```python
from build123d import *

# Parameters (mm, degrees)
F1_DEPTH  = 12.7
F2_R      = 6.35
F3_DEPTH  = 31.242
F4_W      = 6.35
F4_H      = 38.1
F5_DEPTH  = 38.1
F7_DEPTH  = 61.468
F9_DEPTH  = 25.4
F10_R     = 3.175
F11_DEPTH = 50.8


with BuildPart() as f1:
    # F0 (on Top) → F1 (new body)
    with BuildSketch(Plane.XY):
        with BuildLine():
            Line((12.7, -30.8671), (12.697872, 45.100048))
            ThreePointArc((12.697872, 45.100048), (-0.230077, 58.03046), (-12.681114, 44.640199))
            Line((-12.681114, 44.640199), (-12.681114, -30.175112))
            Line((-12.681114, -30.175112), (-12.681114, -31.559801))
            ThreePointArc((-12.681114, -31.559801), (0.346479, -43.562729), (12.7, -30.8671))
        make_face()
        with BuildLine():
            Line((-12.681114, -31.559801), (-12.681114, -30.175112))
            ThreePointArc((-12.681114, -30.175112), (-12.7, -30.867456), (-12.681114, -31.559801))
        make_face()
    extrude(amount=F1_DEPTH)

    # F2 (on face) → F3 (cut)
    with BuildSketch(Plane.XY.offset(12.7)):
        with Locations((0, -30.867456)):
            Circle(F2_R)
        with Locations((0, 45.332544)):
            Circle(F2_R)
    extrude(amount=-F3_DEPTH, mode=Mode.SUBTRACT)

    # F4 (on face) → F5 (join)
    with BuildSketch(Plane.XY.offset(12.7)):
        with Locations((3.175, 7.232544)):
            Rectangle(F4_W, F4_H)
        with Locations((-3.175, 7.232544)):
            Rectangle(F4_W, F4_H)
    extrude(amount=F5_DEPTH)

    # F6 (on face) → F7 (cut)
    with BuildSketch(Plane.XZ.offset(11.817456)):
        with BuildLine():
            ThreePointArc((-6.35, 44.45), (-4.490128, 48.940128), (0, 50.8))
            Line((0, 50.8), (-6.35, 50.8))
            Line((-6.35, 50.8), (-6.35, 44.45))
        make_face()
        with BuildLine():
            ThreePointArc((0, 50.8), (4.490128, 48.940128), (6.35, 44.45))
            Line((6.35, 44.45), (6.35, 50.8))
            Line((6.35, 50.8), (0, 50.8))
        make_face()
    extrude(amount=-F7_DEPTH, mode=Mode.SUBTRACT)

    # F8 (on face) → F9 (cut)
    with BuildSketch(Plane.YZ.offset(6.35)):
        with BuildLine():
            Line((-2.292456, 44.45), (-2.292456, 28.575))
            ThreePointArc((-2.292456, 28.575), (7.32078, 19.050409), (16.755909, 28.751465))
            Line((16.755909, 28.751465), (16.755909, 53.781159))
            Line((16.755909, 53.781159), (-2.292456, 53.781159))
            Line((-2.292456, 53.781159), (-2.292456, 44.45))
        make_face()
    extrude(amount=-F9_DEPTH, mode=Mode.SUBTRACT)

    # F10 (on face) → F11 (cut)
    with BuildSketch(Plane.XZ.offset(11.817456)):
        with Locations((0, 44.45)):
            Circle(F10_R)
    extrude(amount=-F11_DEPTH, mode=Mode.SUBTRACT)


solid = f1.part
```
Source: CAD feature listing. Evaluate the final solid. Frame: model axes, mm. A direction names the side the tool comes from. Round coordinates to 2 decimals unless told otherwise and drop trailing zeros. Loops run counter-clockwise (first coordinate to the right, second up) from the corner with the lowest first, then second, coordinate; pieces in that order, holes last. Notation, with made-up numbers: M -31.75,82 L 1.25,82 A18 cw 1.25,101 Z; hole C -17,15 d7. An arc over 180 degrees is marked long. Use a Markdown table: item, result. Add a question column.
1. Mould query, pull axis X, two halves, no side actions, for faces 1 (the cylindrical face through (-0.83, 51.63, 6.44)), 2 (the flat face through (-6.35, 7, 18)), 3 (the flat face through (0, 26.283, 31)). Classes: pulls with the +X half, pulls with the -X half, needs draft (parallel to the pull), parting line crosses it, or undercut.
2. Section query D-D on x = 7.5. Return the cut outline in (y, z), then the cut area to 3 significant figures.
3. Reachability of faces 4 (the flat face through (0, -11.817, 31)), 5 (the flat face through (6.35, 7, 18)), 6 (the flat face through (0, 16.756, 37)) from +Z, -Z, +X, -X, +Y, -Y: full face, straight path, thin tool, end or side. Return the list, or none.
4. Line query: line 1 (Y direction, x = -2, z = 48.5); line 2 (Y direction, x = 2, z = 12.5); line 3 (X direction, y = -8.5, z = 3). Output: solid intervals per line, ascending.
5. Section query C-C on y = 21.5. Return the cut outline in (x, z) (3 decimals).
6. Section query B-B on y = 47.5. Return the cut outline in (x, z).
7. Section query A-A on z = 32.5. Return the cut outline in (x, y).
8. Contact query for flat-ended pins moving along their axis: P1, Ø4, axis at x = 0, z = 35.5, coming from the -Y side; P2, Ø6.5, axis at y = 21.5, z = 6.5, coming from the -X side; P3, Ø12, axis at x = -8.5, z = 17.5, coming from the -Y side. Output: stop coordinate, or through.
Reported:
| question | item | result |
|---|---|---|
| 1 | face 1 | undercut |
| 1 | face 2 | pulls with the -X half |
| 1 | face 3 | needs draft |
| 2 | outline | M -41.12,0 L 55.58,0 L 55.58,12.7 L -41.12,12.7 Z |
| 2 | area | 1,230 mm² |
| 3 | face 4 | +Z, +X, -X, -Y |
| 3 | face 5 | +Z, +X, +Y, -Y |
| 3 | face 6 | +Z, +X, -X |
| 4 | line 1 | y = -11.82 to -2.29, 16.76 to 26.28 |
| 4 | line 2 | y = -43.41 to -36.89, -24.84 to 39.31, 51.36 to 57.87 |
| 4 | line 3 | x = -12.68 to 12.7 |
| 5 | outline | M -12.681,0 L 12.699,0 L 12.699,12.7 L 6.35,12.7 L 6.35,44.45 A6.35 ccw -6.35,44.45 L -6.35,12.7 L -12.681,12.7 Z; hole C 0,44.45 d6.35 |
| 6 | outline | M -12.51,0 L -5.97,0 L -5.97,12.7 L -12.51,12.7 Z; M 5.97,0 L 12.51,0 L 12.51,12.7 L 5.97,12.7 Z |
| 7 | outline | M -6.35,-11.82 L 6.35,-11.82 L 6.35,-2.29 L -6.35,-2.29 Z; M -6.35,16.76 L 6.35,16.76 L 6.35,26.28 L -6.35,26.28 Z |
| 8 | P1 | stops at y = -11.82 |
| 8 | P2 | stops at x = -12.68 |
| 8 | P3 | stops at y = -42.58 |
